Here's how the part is built. I have some questions about the finished solid (model axes, mm). A direction names the side the tool comes from. Round coordinates to 2 decimals unless told otherwise and drop trailing zeros. Write each loop counter-clockwise with the first axis right and the second up, starting at its lowest first coordinate (ties: lowest second). Pieces come first, ordered by that corner, then holes. Notation, with made-up numbers: (23.5, -35) - (49.5, -35) arc R15 cw to (49.5, -28) - close; hole circle Ø4 at (73.25, -24.5). An arc over 180 degrees is marked (long way). Write item = value, one per line. Start each with the question number.
Item 1: Which directions (+Z, -Z, +X, -X, +Y, -Y) give clear straight access to the entire face, cutting with the end or side of a thin tool? Please do faces 1 (the face through (-58.99, 6.04, 74.82)), 2 (the face through (53.086, 7, 75)), 3 (the face through (-55, 12.7, -12)).
Item 2: If we section it at B-B (x = 9): Please give me the cut outline in (y, z) (3 decimals), and give its area (3 significant figures).
Item 3: Thinking about a two-plate mould opening in X: for faces 4 (the face through (-48.132, 3.139, -74.635)), 5 (the face through (-55, 0, -12)), 6 (the face through (49, 1.27, 75)), which applies, pulls with the +X half, pulls with the -X half, needs draft (parallel to the pull), parting line crosses it, or undercut?
Item 4: If we section it at A-A (z = -23): Please give me the cut outline in (x, y) (3 decimals), and give its area (3 significant figures).
Item 5: For P1, Ø4.5, axis at x = -36.5, y = 9.5, coming from the +Z side; P2, Ø2.5, axis at x = -59.5, z = 76, coming from the -Y side; P3, Ø5, axis at x = -50, z = 76, coming from the -Y side, each with a flat end and sliding along its axis, tell me the tip position at first contact or that it passes through.
Item 6: If I drill on line 1 along X through (y, z) = (10, -32.5) (3 decimals); line 2 along Z through (x, y) = (29, 3.5); line 3 along Z through (x, y) = (-38, 5), over which ranges is the centre line in solid material (lowest first)? Write a range as [from, to].
```python
from build123d import *

# Parameters (mm, degrees)
SKETCH2_W           = 133.35
SKETCH2_H           = 160.866666666
SKETCH2_W_2         = 107.95
SKETCH2_H_2         = 135.466666666
BOSS_EXTRUDE1_DEPTH = 12.7
CUT_EXTRUDE1_DEPTH  = 6.35
CHAMFER1_SIZE       = 0.635
CHAMFER3_SIZE       = 3.81
SKETCH5_W           = 8.89
SKETCH5_H           = 11.43
CUT_EXTRUDE2_DEPTH  = 10.16
SKETCH6_W           = 8.89
SKETCH6_H           = 11.43
CUT_EXTRUDE3_DEPTH  = 10.16
CHAMFER4_SIZE       = 3.175


with BuildPart() as part:
    # Sketch2 → Boss-Extrude1 (new body)
    with BuildSketch(Plane(origin=(0, 0, 0), x_dir=(1, 0, 0), z_dir=(0, 1, 0))):
        Rectangle(SKETCH2_W, SKETCH2_H)
        Rectangle(SKETCH2_W_2, SKETCH2_H_2, mode=Mode.SUBTRACT)
    extrude(amount=BOSS_EXTRUDE1_DEPTH)

    # Sketch4 → Cut-Extrude1 (cut)
    with BuildSketch(Plane(origin=(0, 0, 0), x_dir=(1, 0, 0), z_dir=(0, 1, 0))):
        Polygon((-63.5, 76.2), (-60.325, 79.375), (-57.15, 76.2), (-60.325, 73.025), align=None)
        Polygon((-52.916666667, 76.2), (-49.741666667, 79.375), (-46.566666667, 76.2), (-49.741666667, 73.025), align=None)
        Polygon((57.15, 76.2), (60.325, 79.375), (63.5, 76.2), (60.325, 73.025), align=None)
        Polygon((57.15, -76.2), (60.325, -73.025), (63.5, -76.2), (60.325, -79.375), align=None)
        Polygon((-52.916666667, -76.2), (-49.741666667, -73.025), (-46.566666667, -76.2), (-49.741666667, -79.375), align=None)
        Polygon((-63.5, -76.2), (-60.325, -73.025), (-57.15, -76.2), (-60.325, -79.375), align=None)
    extrude(amount=CUT_EXTRUDE1_DEPTH, mode=Mode.SUBTRACT)

    # Chamfer1
    chamfer1_edges = [part.edges().sort_by_distance(p)[0] for p in [
        (-61.9125, 0, 77.7875),
        (-58.7375, 0, 77.7875),
        (-58.7375, 0, 74.6125),
        (-61.9125, 0, 74.6125),
        (-61.9125, 6.35, 77.7875),
        (-58.7375, 6.35, 77.7875),
        (-58.7375, 6.35, 74.6125),
        (-61.9125, 6.35, 74.6125),
        (-51.329166667, 0, 77.7875),
        (-52.916666667, 3.175, 76.2),
        (-48.154166667, 0, 77.7875),
        (-48.154166667, 0, 74.6125),
        (-51.329166667, 0, 74.6125),
        (-49.741666667, 3.175, 73.025),
        (-51.329166667, 6.35, 77.7875),
        (-48.154166667, 6.35, 77.7875),
        (-48.154166667, 6.35, 74.6125),
        (-51.329166667, 6.35, 74.6125),
        (58.7375, 0, 77.7875),
        (61.9125, 0, 77.7875),
        (61.9125, 0, 74.6125),
        (58.7375, 0, 74.6125),
        (58.7375, 6.35, 77.7875),
        (61.9125, 6.35, 77.7875),
        (61.9125, 6.35, 74.6125),
        (58.7375, 6.35, 74.6125),
        (58.7375, 0, -74.6125),
        (61.9125, 0, -74.6125),
        (61.9125, 0, -77.7875),
        (58.7375, 0, -77.7875),
        (58.7375, 6.35, -74.6125),
        (61.9125, 6.35, -74.6125),
        (61.9125, 6.35, -77.7875),
        (58.7375, 6.35, -77.7875),
        (-51.329166667, 0, -74.6125),
        (-48.154166667, 0, -74.6125),
        (-48.154166667, 0, -77.7875),
        (-51.329166667, 0, -77.7875),
        (-51.329166667, 6.35, -74.6125),
        (-48.154166667, 6.35, -74.6125),
        (-48.154166667, 6.35, -77.7875),
        (-51.329166667, 6.35, -77.7875),
        (-61.9125, 0, -74.6125),
        (-58.7375, 0, -74.6125),
        (-58.7375, 0, -77.7875),
        (-61.9125, 0, -77.7875),
        (-61.9125, 6.35, -74.6125),
        (-58.7375, 6.35, -74.6125),
        (-58.7375, 6.35, -77.7875),
        (-61.9125, 6.35, -77.7875),
    ]]
    chamfer(chamfer1_edges, length=CHAMFER1_SIZE)

    # Chamfer3
    chamfer3_edges = [part.edges().sort_by_distance(p)[0] for p in [
        (0, 12.7, -80.433333333),
        (0, 12.7, 80.433333333),
    ]]
    chamfer(chamfer3_edges, length=CHAMFER3_SIZE)

    # Sketch5 → Cut-Extrude2 (cut)
    with BuildSketch(Plane.XY.offset(80.433333333)):
        with Locations((-38.0365, 6.985)):
            Rectangle(SKETCH5_W, SKETCH5_H)
        with Locations((48.641, 6.985)):
            Rectangle(SKETCH5_W, SKETCH5_H)
    extrude(amount=-CUT_EXTRUDE2_DEPTH, mode=Mode.SUBTRACT)

    # Sketch6 → Cut-Extrude3 (cut)
    with BuildSketch(Plane(origin=(0, 0, -80.433333333), x_dir=(-1, 0, 0), z_dir=(0, 0, -1))):
        with Locations((38.0365, 6.985)):
            Rectangle(SKETCH6_W, SKETCH6_H)
        with Locations((-48.641, 6.985)):
            Rectangle(SKETCH6_W, SKETCH6_H)
    extrude(amount=-CUT_EXTRUDE3_DEPTH, mode=Mode.SUBTRACT)

    # Chamfer4
    chamfer4_edges = [part.edges().sort_by_distance(p)[0] for p in [
        (0, 0, -67.733333333),
        (0, 0, 67.733333333),
    ]]
    chamfer(chamfer4_edges, length=CHAMFER4_SIZE)


solid = part.part
```
Reply:
q1.face_1 = -Y
q1.face_2 = +Z, +Y
q1.face_3 = +Z, -Z, +X, -X, +Y
q2.outline = (0, -80.433) - (8.89, -80.433) - (12.7, -76.623) - (12.7, -67.733) - (3.175, -67.733) - (0, -70.908) - close; (0, 70.908) - (3.175, 67.733) - (12.7, 67.733) - (12.7, 76.623) - (8.89, 80.433) - (0, 80.433) - close
q2.area = 298 mm2
q3.face_4 = undercut
q3.face_5 = needs draft
q3.face_6 = undercut
q4.outline = (-66.675, 0) - (-53.975, 0) - (-53.975, 12.7) - (-66.675, 12.7) - close; (53.975, 0) - (66.675, 0) - (66.675, 12.7) - (53.975, 12.7) - close
q4.area = 323 mm2
q5.P1 = 70.27
q5.P2 = 5.99
q5.P3 = 0.06
q6.line_1 = [-66.675, -53.975], [53.975, 66.675]
q6.line_2 = [-80.43, -67.73], [67.73, 80.43]
q6.line_3 = [-70.27, -67.73], [67.73, 70.27]
